Autodesk Inventor part; units mm, degrees
ref_plane "YZ Plane" through (0, 0, 0) normal (1, 0, 0) x (0, 1, 0)
ref_plane "XZ Plane" through (0, 0, 0) normal (0, 1, 0) x (-1, 0, 0)
ref_plane "XY Plane" through (0, 0, 0) normal (0, 0, 1) x (1, 0, 0)
sketch "Sketch2" plane through (0, 0, 0) normal (0, 0, 1) x (1, 0, 0)
  line L0 (-46, 10) -> (46, 10)
  line L1 (47, 9) -> (47, -9)
  line L2 (46, -10) -> (-46, -10)
  line L3 (-47, -9) -> (-47, 9)
  line L4 (-47, 10) -> (47, -10) construction
  line L5 (47, 10) -> (-47, -10) construction
  line L6 (45, 8) -> (-45, 8)
  line L7 (-45, 8) -> (-45, -8)
  line L8 (-45, -8) -> (45, -8)
  line L9 (45, -8) -> (45, 8)
  line L10 (48, 11) -> (-48, 11)
  line L11 (-48, 11) -> (-48, -11)
  line L12 (-48, -11) -> (48, -11)
  line L13 (48, -11) -> (48, 11)
  arc A0 (47, 9) -> (46, 10) centre (46, 9) ccw
  arc A1 (46, -10) -> (47, -9) centre (46, -9) ccw
  arc A2 (-47, -9) -> (-46, -10) centre (-46, -9) ccw
  arc A3 (-46, 10) -> (-47, 9) centre (-46, 9) ccw
  point P0 (0, 0)
  dimension "d0" = 94
  dimension "d1" = 20
  dimension "d2" = 2
  dimension "d3" = 1
  dimension "d10" = 1
  dimension "d40" = 90
extrude "Extrusion1" add sketch "Sketch2" along normal blind 1 contours L0 A0 L1 A1 L2 A2 L3 A3 | L9 L8 L7 L6 | L13 L12 L11 L10
extrude "Extrusion2" add sketch "Sketch2" along normal blind 7 contours L13 L12 L11 L10
extrude "Extrusion3" add sketch "Sketch2" along normal blind 4 contours L9 L8 L7 L6
sketch "Sketch4" plane through (-48, -11, 0) normal (0, -1, 0) x (1, 0, 0)
  circle A0 centre (22.1132, 5) radius 0.5
  circle A1 centre (29.8868, 5) radius 0.5
  circle A2 centre (44.1132, 5) radius 0.5
  circle A3 centre (51.8842, 5) radius 0.5
  circle A4 centre (66.1132, 5) radius 0.5
  circle A5 centre (73.8868, 5) radius 0.5
  line L0 (0, 6) -> (96, 6)
  line L1 (96, 7) -> (0, 7)
  line L2 (22.1132, 2) -> (22.1132, 2)
  line L3 (22.6132, 2.5) -> (22.6132, 8)
  line L4 (22.6132, 8) -> (21.6132, 8)
  line L5 (21.6132, 8) -> (21.6132, 2.5)
  line L6 (21.6132, 2) -> (22.6132, 8) construction
  line L7 (22.6132, 2) -> (21.6132, 8) construction
  line L8 (29.8868, 2) -> (29.8868, 2)
  line L9 (30.3868, 2.5) -> (30.3868, 8)
  line L10 (30.3868, 8) -> (29.3868, 8)
  line L11 (29.3868, 8) -> (29.3868, 2.5)
  line L12 (29.3868, 2) -> (30.3868, 8) construction
  line L13 (30.3868, 2) -> (29.3868, 8) construction
  line L14 (44.1132, 2) -> (44.1132, 2)
  line L15 (44.6132, 2.5) -> (44.6132, 8)
  line L16 (44.6132, 8) -> (43.6132, 8)
  line L17 (43.6132, 8) -> (43.6132, 2.5)
  line L18 (43.6132, 2) -> (44.6132, 8) construction
  line L19 (44.6132, 2) -> (43.6132, 8) construction
  line L20 (51.8842, 2) -> (51.8842, 2)
  line L21 (52.3842, 2.5) -> (52.3842, 8)
  line L22 (52.3842, 8) -> (51.3842, 8)
  line L23 (51.3842, 8) -> (51.3842, 2.5)
  line L24 (51.3842, 2) -> (52.3842, 8) construction
  line L25 (52.3842, 2) -> (51.3842, 8) construction
  line L26 (66.1132, 2) -> (66.1132, 2)
  line L27 (65.6132, 2.5) -> (65.6132, 8)
  line L28 (65.6132, 8) -> (66.6132, 8)
  line L29 (66.6132, 8) -> (66.6132, 2.5)
  line L30 (66.6132, 2) -> (65.6132, 8) construction
  line L31 (65.6132, 2) -> (66.6132, 8) construction
  line L32 (73.8868, 2) -> (73.8868, 2)
  line L33 (73.3868, 2.5) -> (73.3868, 8)
  line L34 (73.3868, 8) -> (74.3868, 8)
  line L35 (74.3868, 8) -> (74.3868, 2.5)
  line L36 (74.3868, 2) -> (73.3868, 8) construction
  line L37 (73.3868, 2) -> (74.3868, 8) construction
  arc A6 (21.6132, 2.5) -> (22.1132, 2) centre (22.1132, 2.5) ccw
  arc A7 (22.1132, 2) -> (22.6132, 2.5) centre (22.1132, 2.5) ccw
  arc A8 (29.3868, 2.5) -> (29.8868, 2) centre (29.8868, 2.5) ccw
  arc A9 (29.8868, 2) -> (30.3868, 2.5) centre (29.8868, 2.5) ccw
  arc A10 (43.6132, 2.5) -> (44.1132, 2) centre (44.1132, 2.5) ccw
  arc A11 (44.1132, 2) -> (44.6132, 2.5) centre (44.1132, 2.5) ccw
  arc A12 (51.3842, 2.5) -> (51.8842, 2) centre (51.8842, 2.5) ccw
  arc A13 (51.8842, 2) -> (52.3842, 2.5) centre (51.8842, 2.5) ccw
  arc A14 (65.6132, 2.5) -> (66.1132, 2) centre (66.1132, 2.5) ccw
  arc A15 (66.1132, 2) -> (66.6132, 2.5) centre (66.1132, 2.5) ccw
  arc A16 (73.3868, 2.5) -> (73.8868, 2) centre (73.8868, 2.5) ccw
  arc A17 (73.8868, 2) -> (74.3868, 2.5) centre (73.8868, 2.5) ccw
  point P0 (96, 0)
  point P1 (69, 6)
  point P2 (71, 6)
  point P3 (49, 6)
  point P4 (47, 6)
  point P5 (27, 6)
  point P6 (25, 6)
  point P7 (73.8868, 2)
  point P8 (66.1132, 2)
  point P9 (51.8842, 2)
  point P10 (44.1132, 2)
  point P11 (29.8868, 2)
  point P12 (22.1132, 2)
  dimension "d59" = 1
  dimension "d60" = 1
  dimension "d61" = 1
  dimension "d62" = 1
  dimension "d63" = 1
  dimension "d64" = 1
  dimension "d65" = 1
  dimension "d66" = 6
  dimension "d67" = 1
  dimension "d68" = 6
  dimension "d69" = 1
  dimension "d70" = 6
  dimension "d71" = 1
  dimension "d72" = 6
  dimension "d73" = 1
  dimension "d74" = 6
  dimension "d75" = 1
  dimension "d76" = 6
  dimension "d81" = 0.5
sketch "Sketch3" plane through (0, -11, 4) normal (0, -1, 0) x (1, 0, 0)
  line L0 (-53.1158, -2.5) -> (46.8842, -2.5) construction
  line L1 (43, -1.5) -> (23, -1.5) construction
  line L2 (23, -1.5) -> (23, 3.5) construction
  line L3 (23, 3.5) -> (43, 3.5) construction
  line L4 (43, 3.5) -> (43, -1.5) construction
  line L5 (23, -1.5) -> (23, 3.7137) construction
  line L6 (43, -1.5) -> (40.1132, 3.5) construction
  line L7 (46.8842, -2.5) -> (46.8842, 3.2735) construction
  line L8 (23, -1.5) -> (25.8868, 3.5) construction
  line L9 (23, -1.5) -> (23, 3.1279) construction
  line L10 (21, -1.5) -> (18.1132, 3.5) construction
  line L11 (1, 3.5) -> (21, 3.5) construction
  line L12 (1, -1.5) -> (3.8868, 3.5) construction
  line L13 (-1, -1.5) -> (-3.8868, 3.5) construction
  line L14 (-21, 3.5) -> (-1, 3.5) construction
  line L15 (-21, -1.5) -> (-18.1132, 3.5) construction
  line L16 (-23, -1.5) -> (-25.8868, 3.5) construction
  line L17 (-43, 3.5) -> (-23, 3.5) construction
  line L18 (-43, -1.5) -> (-40.1132, 3.5) construction
  line L19 (43, 3.5) -> (-43, 3.5) construction
  line L20 (0, 3.5) -> (0, 3.5) construction
  circle A0 centre (-25.8868, -1.5) radius 0.5
  circle A1 centre (-18.1132, -1.5) radius 0.5
  circle A2 centre (-3.8868, -1.5) radius 0.5
  circle A3 centre (3.8842, -1.5) radius 0.5
  circle A4 centre (18.1132, -1.5) radius 0.5
  circle A5 centre (25.8868, -1.5) radius 0.5
  line L21 (-45, 0) -> (-45, 0)
  line L22 (45, 0) -> (45, 0)
  line L23 (-48, -4) -> (-48, -4)
  line L24 (-48, -1.5) -> (48, -1.5)
  line L25 (48, -4) -> (48, -4)
  line L26 (48, -4) -> (48, 3)
  point P0 (3.8842, 2.5)
  point P1 (25.8868, -1.5)
  point P2 (48, -0.5)
  dimension "d45" = 20
  dimension "d46" = 5
  dimension "d47" = 30
  dimension "d48" = 30
  dimension "d49" = 22
  dimension "d52" = 0
  dimension "d53" = 1
  dimension "d54" = 1
  dimension "d55" = 1
  dimension "d56" = 1
  dimension "d57" = 1
  dimension "d58" = 1
  dimension "d82" = 1
extrude "Extrusion4" cut sketch "Sketch4" against normal blind 2 contours A0 | L3 A7 A6 L5 A0 | A0 L5 L0 L3 | L0 L5 L1 L3 | L11 L1 L9 L0 | L0 L9 A1 L11 | L1 L5 L4 L3 | L11 L10 L9 L1 | A1 | A1 L9 A9 A8 L11 | L17 L1 L15 L0 | L0 L15 A2 L17 | L17 L16 L15 L1 | A2 | A2 L15 A11 A10 L17 | L23 L1 L21 L0 | L0 L21 A3 L23 | L23 L22 L21 L1 | A3 | A3 L21 A13 A12 L23 | L27 L1 L29 L0 | L0 L29 A4 L27 | A4 | A4 L29 A15 A14 L27 | L27 L28 L29 L1 | L33 L1 L35 L0 | L0 L35 A5 L33 | A5 | A5 L35 A17 A16 L33 | L33 L34 L35 L1
extrude "Extrusion5" cut sketch "Sketch3" against normal blind 10
properties part number "sdm_finger_eit_chamber_mould_horizontal_e_holes"
Model file for the job. Use its own axes, mm. A direction names the side the tool comes from. Coordinates: 2 decimals unless noted, no trailing zeros. Order: outer loops, then holes, each group sorted by start corner. A loop starts at its lowest first (then second) coordinate and runs counter-clockwise, first axis right, second up. Notation, with made-up numbers: M -35,64.25 L -5,64.25 A12 ccw -5,78.25 Z; hole C 74,79.25 d4. An arc over 180 degrees is marked long. Return JSON: item names as keys, results as strings.
1. Pull direction X, two halves, no side cores. Call faces 3 (the face through (48, 0, 3)), 4 (the face through (-1, 0, 0)), 5 (the face through (-0.2, 8.2, 1)): +X half, -X half, draft (parallel to the pull), parting line (faces both ways), or undercut.
Ans:
{"face 3": "+X half", "face 4": "draft", "face 5": "undercut"}
2. Tool access for faces 1 (the face through (1, -10, 4)), 2 (the face through (-48, 0, 3)): list every direction of +Z, -Z, +X, -X, +Y, -Y with a clear straight run to the whole face (end or side of a thin tool).
Ans:
{"face 1": "+Z", "face 2": "+Z, -Z, -X, +Y, -Y"}
3. Drill centre lines: probe 1 along Y at (x, z) = (5, 3); probe 2 along X at (y, z) = (-0.75, 3.5); probe 3 along X at (y, z) = (-6.25, 6). Where is each one in solid material? Low to high.
Ans:
{"probe 1": "-11 to -10, -8 to 8, 10 to 11", "probe 2": "-48 to -47, -45 to 45, 47 to 48", "probe 3": "-48 to -47, 47 to 48"}
4. Flat gauge pins, fed straight in: pin 1 (10 mm diameter, centred on x = -9.5, y = 1.5, fed in from +Z); pin 2 (0.5 mm diameter, centred on x = -4, z = 2.5, fed in from -Y). Where does each tip first touch, or does it go through?
Ans:
{"pin 1": "z = 4", "pin 2": "y = -1"}
5. Saw through at B-B (x = 32.5). Give the cut face in (y, z).
Ans:
{"outline": "M -11,0 L 11,0 L 11,7 L 10,7 L 10,1 L 8,1 L 8,4 L -8,4 L -8,1 L -10,1 L -10,7 L -11,7 Z"}
6. Saw through at A-A (y = -3). Give the cut face in (x, z).
Ans:
{"outline": "M -48,0 L 48,0 L 48,7 L 47,7 L 47,1 L 45,1 L 45,4 L -45,4 L -45,1 L -47,1 L -47,7 L -48,7 Z; hole C -25.89,2.5 d1; hole C -18.11,2.5 d1; hole C -3.89,2.5 d1; hole C 3.88,2.5 d1; hole C 18.11,2.5 d1; hole C 25.89,2.5 d1"}
7. Saw through at C-C (y = 1.5). Give the cut face in (x, z), and give its area (3 significant figures).
Ans:
{"outline": "M -48,0 L 48,0 L 48,7 L 47,7 L 47,1 L 45,1 L 45,4 L -45,4 L -45,1 L -47,1 L -47,7 L -48,7 Z", "area": "378 mm^2"}
